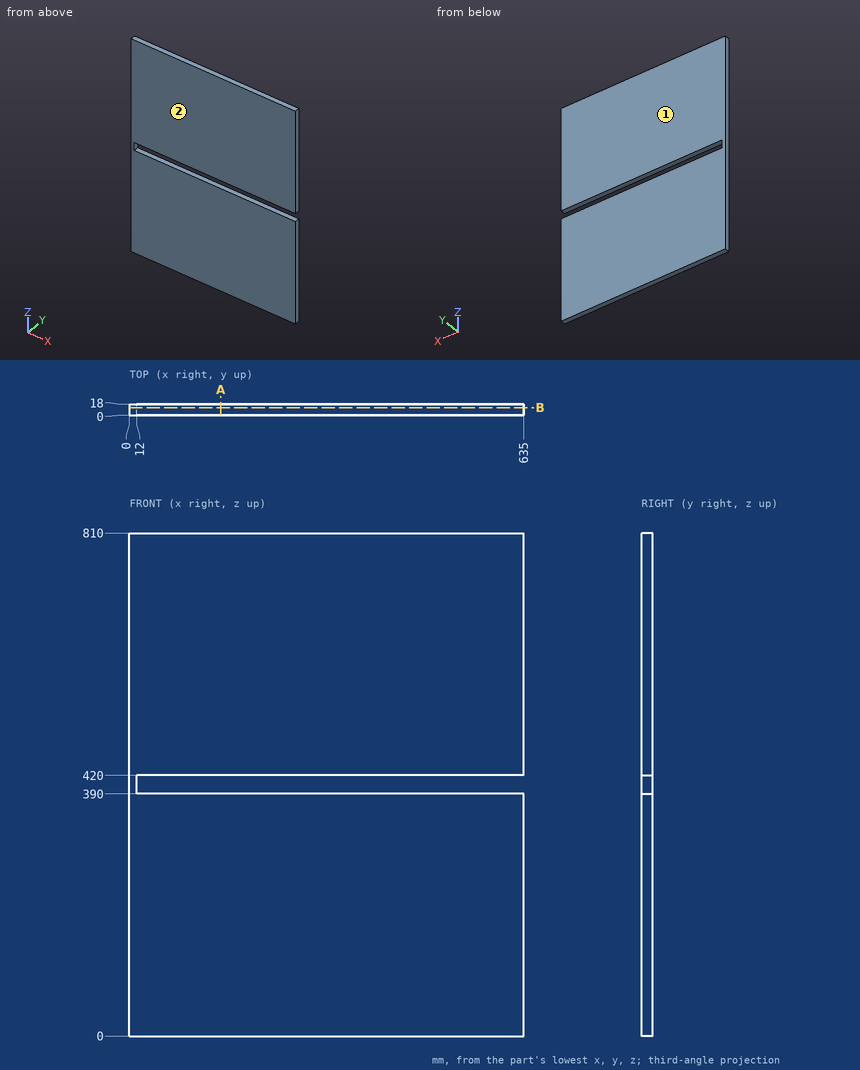
The drawing under review shows one solid part. Ordinate dimensions are in mm from its lowest x, y, z. Coordinates: 2 decimals unless noted, no trailing zeros. Write each loop counter-clockwise with the first axis right and the second up, starting at its lowest first coordinate (ties: lowest second). Pieces come first, ordered by that corner, then holes. Notation, with made-up numbers: (11.25, 69.5) - (40.25, 69.5) arc R6 cw to (40.25, 74.5) - close; hole circle Ø2 at (52.5, 56). An arc over 180 degrees is marked (long way). Answer in a Markdown table with one row per item. Add a question column.
Q1. We need section B-B, the plane y = 12. State the section outline as (x, z) points.
Q2. For probe 1 along Z at (x, y) = (29, 4.75), list the stretches that pass through material, from the lowest coordinate up.
Q3. For P1, Ø10, axis at x = 399, y = 13, coming from the -Z side, flat-tipped, find the tip position at first contact; note if it passes through.
Q4. We need section A-A, the plane x = 147.5. State the section outline as (y, z) points.
Q5. Draft analysis for pull direction Y (two halves, no side actions). For the marked faces 1 and 2, state which applies: +Y half, -Y half, draft (parallel to the pull), parting line (faces both ways), or undercut.
Answer list:
| question | item | result |
|---|---|---|
| 1 | outline | (0, 0) - (635, 0) - (635, 390) - (12, 390) - (12, 420) - (635, 420) - (635, 810) - (0, 810) - close |
| 2 | probe 1 | z = 0 to 390, 420 to 810 |
| 3 | P1 | stops at z = 0 |
| 4 | outline | (0, 0) - (18, 0) - (18, 390) - (0, 390) - close; (0, 420) - (18, 420) - (18, 810) - (0, 810) - close |
| 5 | face 1 | +Y half |
| 5 | face 2 | -Y half |
